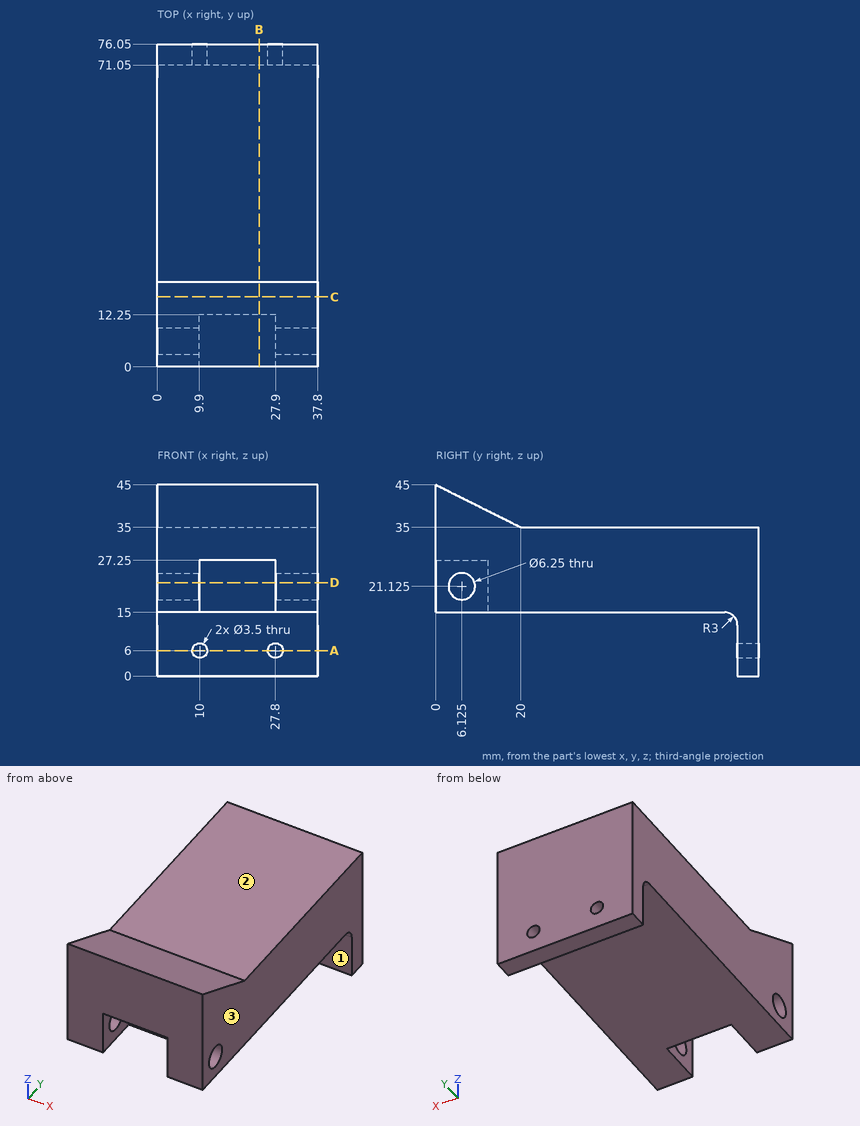
Verification items for this drawing (mm, ordinates from the low corner). A direction names the side the tool comes from. Give positions to 0.01 mm unless a question says otherwise; leave off trailing zeros. Loops run counter-clockwise (first coordinate to the right, second up) from the corner with the lowest first, then second, coordinate; pieces in that order, holes last. Notation, with made-up numbers: M 17,82 L 25,82 A9 cw 25,90 Z; hole C 88,49 d6. An arc over 180 degrees is marked long. Write each question's results on one line, items separated by ' | '.
1) Thickness scan on line 1 (X direction, y = 72, z = 6); line 2 (Z direction, x = 33.5, y = 30); line 3 (Y direction, x = 12.5, z = 24). Record the ranges inside material, lowest first.
Answers follow:
line 1: 0 to 8.25, 11.75 to 26.05, 29.55 to 37.8 | line 2: 15 to 35 | line 3: 12.25 to 76.05
2) Tool access check on the marked faces 1, 2 and 3. Record the directions out of +Z, -Z, +X, -X, +Y, -Y that give a thin tool (end or side, any length) a straight path to the whole face; none if there is none.
Answers follow:
face 1: -Z, +X, -X, -Y | face 2: +Z, +X, -X, +Y | face 3: +Z, -Z, +X, +Y, -Y
3) Section check C-C, the plane y = 16.5. Record the boundary of the cut face in (x, z), plus the area to 3 significant figures.
Answers follow:
outline: M 0,15 L 37.8,15 L 37.8,36.75 L 0,36.75 Z | area: 822 mm2
4) Section check B-B, the plane x = 24. Record the boundary of the cut face in (y, z), plus the area to 3 significant figures.
Answers follow:
outline: M 0,27.25 L 12.25,27.25 L 12.25,15 L 68.05,15 A3 cw 71.05,12 L 71.05,0 L 76.05,0 L 76.05,35 L 20,35 L 0,45 Z | area: 1,550 mm2
5) Section check D-D, the plane z = 22. Record the boundary of the cut face in (x, y) (3 decimals).
Answers follow:
outline: M 0,0 L 9.9,0 L 9.9,3.125 L 0,3.125 Z; M 0,9.125 L 9.9,9.125 L 9.9,12.25 L 27.9,12.25 L 27.9,9.125 L 37.8,9.125 L 37.8,76.05 L 0,76.05 Z; M 27.9,0 L 37.8,0 L 37.8,3.125 L 27.9,3.125 Z
6) Section check A-A, the plane z = 6. Record the boundary of the cut face in (x, y), plus the area to 3 significant figures.
Answers follow:
outline: M 0,71.05 L 8.25,71.05 L 8.25,76.05 L 0,76.05 Z; M 11.75,71.05 L 26.05,71.05 L 26.05,76.05 L 11.75,76.05 Z; M 29.55,71.05 L 37.8,71.05 L 37.8,76.05 L 29.55,76.05 Z | area: 154 mm2
7) Gauge pin test, flat ends, axial feed: pin 1 (1.5 mm diameter, centred on x = 28.5, z = 37, fed in from +Y); pin 2 (13.5 mm diameter, centred on x = 17.5, y = 8.5, fed in from -Z); pin 3 (6 mm diameter, centred on x = 30.5, y = 51, fed in from +Z). Record the tip position at first contact, or that the pin passes through.
Answers follow:
pin 1: y = 17.5 | pin 2: z = 15 | pin 3: z = 35
